Geometry: final body of the model. Coordinates: model frame, mm. A direction names the side the tool comes from. Give positions to 0.01 mm unless a question says otherwise; leave off trailing zeros. Loops run counter-clockwise (first coordinate to the right, second up) from the corner with the lowest first, then second, coordinate; pieces in that order, holes last. Notation, with made-up numbers: (29, 51) -> (64, 51) arc R18 ccw to (64, 59) -> close; hole circle Ø8 at (40, 86). An arc over 180 degrees is marked (long way). One line per item, written item: value. Start each with the question number.
from build123d import *

# Parameters (mm, degrees)
BOSS_EXTRUDE1_DEPTH      = 10.5
BOSS_EXTRUDE2_DEPTH      = 5.08
BOSS_EXTRUDE2_DEPTH_BACK = 1.27
SKETCH3_W                = 20.5486
SKETCH3_H                = 1.0414
BOSS_EXTRUDE3_DEPTH      = 5.08
BOSS_EXTRUDE3_DEPTH_BACK = 1.27
SKETCH4_W                = 20.5486
SKETCH4_H                = 0.508


with BuildPart() as part:
    # Sketch1 → Boss-Extrude1 (new, symmetric)
    with BuildSketch(Plane.XY):
        with BuildLine():
            Line((0, 0), (19.01175011, 0))
            ThreePointArc((19.01175011, 0), (55.726625118, 36.714875008), (19.01175011, 73.429750016))
            Line((19.01175011, 73.429750016), (5.549000018, 73.429750016))
            Line((5.549000018, 73.429750016), (5.549000018, 73.175750016))
            Line((5.549000018, 73.175750016), (19.01175011, 73.175750016))
            ThreePointArc((19.01175011, 73.175750016), (55.472625118, 36.714875008), (19.01175011, 0.254))
            Line((19.01175011, 0.254), (0, 0.254))
            Line((0, 0.254), (0, 0))
        make_face()
    extrude(amount=BOSS_EXTRUDE1_DEPTH, both=True)

    # Sketch3 → Boss-Extrude2 (add, two sides: drawn at the far end of the back side and taken through both)
    with BuildSketch(Plane.ZY.offset(-BOSS_EXTRUDE2_DEPTH_BACK)):
        with Locations((0, -0.4953)):
            Rectangle(SKETCH3_W, SKETCH3_H)
    extrude(amount=BOSS_EXTRUDE2_DEPTH + BOSS_EXTRUDE2_DEPTH_BACK)

    # Sketch4 → Boss-Extrude3 (add, two sides: drawn at the far end of the back side and taken through both)
    with BuildSketch(Plane.ZY.offset(-5.549000018).offset(-BOSS_EXTRUDE3_DEPTH_BACK)):
        with Locations((0, 73.455150016)):
            Rectangle(SKETCH4_W, SKETCH4_H)
    extrude(amount=BOSS_EXTRUDE3_DEPTH + BOSS_EXTRUDE3_DEPTH_BACK)


solid = part.part
Item 1: Section D-D, the plane x = 51.5. Output: boundary loops of the cut face in (y, z).
Item 2: Mould query, pull axis Y, two halves, no side actions, for faces 1 (the face through (3, 73.201, 0)), 2 (the face through (55.718, 35.908, 0.147)), 3 (the face through (-2, -1.016, 0)). Classes: pulls with the +Y half, pulls with the -Y half, needs draft (parallel to the pull), parting line crosses it, or undercut.
Item 3: Ray query, line 1 along Y through (x, z) = (15, -8); line 2 along Y through (x, z) = (37, 0.25); line 3 along Y through (x, z) = (-1.5, 1). Return the intervals inside material, ascending. Write a range as [from, to].
Item 4: Pin query (flat end, axial travel): pin 1 (4 mm diameter, centred on x = 14, z = 5, fed in from +Y); pin 2 (4 mm diameter, centred on x = 45.5, z = -7, fed in from -Y); pin 3 (5.5 mm diameter, centred on x = 7.5, z = -3, fed in from -Y). Return the tip coordinate at first contact, or that it passes through.
Item 5: Section C-C, the plane y = 59. Output: boundary loops of the cut face in (x, z).
Item 6: Section B-B, the plane x = 38.5. Output: boundary loops of the cut face in (y, z).
Item 7: Access query for faces 4 (the face through (10, 0.254, 0)), 5 (the face through (-3, 0.025, 0)), 6 (the face through (4, 73.709, 0)). Directions: +Z, -Z, +X, -X, +Y, -Y. A direction counts if a zero-diameter tool reaches every point of the face in a straight line with its end or side. Return the directions, or none.
Geometry check:
1. outline: (19.61, -10.5) -> (20.16, -10.5) -> (20.16, 10.5) -> (19.61, 10.5) -> close; (53.27, -10.5) -> (53.82, -10.5) -> (53.82, 10.5) -> (53.27, 10.5) -> close
2. face 1: undercut
2. face 2: parting line crosses it
2. face 3: pulls with the -Y half
3. line 1: y = [0, 0.25], [73.18, 73.43]
3. line 2: y = [4.71, 5], [68.43, 68.72]
3. line 3: y = [-1.02, 0.03]
4. pin 1: stops at y = 73.43
4. pin 2: stops at y = 9.36
4. pin 3: stops at y = 0
5. outline: (47.87, -10.5) -> (48.19, -10.5) -> (48.19, 10.5) -> (47.87, 10.5) -> close
6. outline: (5.6, -10.5) -> (5.9, -10.5) -> (5.9, 10.5) -> (5.6, 10.5) -> close; (67.53, -10.5) -> (67.83, -10.5) -> (67.83, 10.5) -> (67.53, 10.5) -> close
7. face 4: +Z, -Z, -X
7. face 5: +Z, -Z, -X, +Y
7. face 6: +Z, -Z, +X, -X, +Y
